Verification items for the finished model (mm, model axes). Face numbers are marked on the shaded views. A direction names the side the tool comes from. Round coordinates to 2 decimals unless told otherwise and drop trailing zeros. Write each loop counter-clockwise with the first axis right and the second up, starting at its lowest first coordinate (ties: lowest second). Pieces come first, ordered by that corner, then holes. Notation, with made-up numbers: M -0.5,28.25 L 42.5,28.25 A10 cw 42.5,47.25 Z; hole C 62.5,54 d1. An arc over 180 degrees is marked long. One line per item, written item: value. Start each with the question number.
Item 1: Gauge pin test, flat ends, axial feed: pin 1 (2 mm diameter, centred on x = -3, y = -4.5, fed in from +Z); pin 2 (2.5 mm diameter, centred on x = -0.5, z = -7.5, fed in from -Y); pin 3 (3 mm diameter, centred on x = -3, z = -7.5, fed in from -Y). Record the tip position at first contact, or that the pin passes through.
Item 2: Section check A-A, the plane y = -8. Record the cut outline in (x, z), then the cut area to 3 significant figures.
Item 3: Section check D-D, the plane y = -9.75. Record the cut outline in (x, z), then the cut area to 3 significant figures.
Item 4: Section check B-B, the plane z = 2. Record the cut outline in (x, y), then the cut area to 3 significant figures.
Item 5: Tool access check on the marked faces 5 and 6. Record the directions out of +Z, -Z, +X, -X, +Y, -Y that give a thin tool (end or side, any length) a straight path to the whole face; none if there is none.
Item 6: Draft check along Y on the marked faces 1, 2, 3 and 4. Enter one of: +Y half, -Y half, draft (parallel to the pull), parting line (faces both ways), or undercut.
Item 7: Thickness scan on probe 1 along Z at (x, y) = (-1, -4.5); probe 2 along Y at (x, z) = (3, -1); probe 3 along Y at (x, z) = (-2.75, -4.5). Record the ranges inside material, lowest first. Write a range as from..to.
Item 8: Section check C-C, the plane x = 1.25. Record the cut outline in (y, z), then the cut area to 3 significant figures.
from build123d import *

# Parameters (mm, degrees)
F1_DEPTH    = 4
F2_T1_DEPTH = 10.764079149
F3_W        = 8
F3_H        = 10
F4_DEPTH    = 7
F5_W        = 8
F5_H        = 2.2
F5_W_2      = 11
F5_H_2      = 2.9
F6_DEPTH    = 25
F7_T1_DEPTH = 18
F7_T3_DEPTH = 17.9874921777
F8_W        = 10.9849025458
F8_H        = 7.8663821071
F9_DEPTH    = 25
F11_DEPTH   = 8
F12_R       = 1


# Not quite as in the source:
# - a fillet or chamfer that OpenCascade refuses, or shapes differently, is made with other operations: its cross-section is extruded or revolved along the edge and cut away or added


with BuildPart() as f1:
    # F0 (on Front) → F1 (new body)
    with BuildSketch(Plane.XZ):
        with BuildLine():
            Line((-1.02606043, 2.8190778624), (-1.3680805733, 3.7587704831))
            ThreePointArc((-1.3680805733, 3.7587704831), (-3.2766081772, 2.2943057454), (-4, 0))
            Line((-4, 0), (-4, -8))
            Line((-4, -8), (-4, -13))
            Line((-4, -13), (4, -13))
            Line((4, -13), (4, -3))
            Line((4, -3), (4, 0))
            ThreePointArc((4, 0), (3.2766081772, 2.2943057454), (1.3680805733, 3.7587704831))
            Line((1.3680805733, 3.7587704831), (1.02606043, 2.8190778624))
            ThreePointArc((1.02606043, 2.8190778624), (0, -3), (-1.02606043, 2.8190778624))
        make_face()
    extrude(amount=F1_DEPTH)

    # F2: fillet of radius 1 on 2 edges, made by hand

    # F2_s2 → F2_t1 (cut)
    with BuildSketch(Plane.XZ.offset(-3.3820395745)):
        with BuildLine():
            ThreePointArc((-2.5427622285, 3.087775939), (-1.6437981614, 3.280553188), (-0.9673790506, 2.6578520976))
            Line((-0.9673790506, 2.6578520976), (-1.3680805733, 3.7587704831))
            ThreePointArc((-1.3680805733, 3.7587704831), (-1.9839937688, 3.4732936423), (-2.5427622285, 3.087775939))
        make_face()
        with BuildLine():
            ThreePointArc((2.5427622285, 3.087775939), (1.6437981614, 3.280553188), (0.9673790506, 2.6578520976))
            Line((0.9673790506, 2.6578520976), (1.3680805733, 3.7587704831))
            ThreePointArc((1.3680805733, 3.7587704831), (1.9839937688, 3.4732936423), (2.5427622285, 3.087775939))
        make_face()
    extrude(amount=F2_T1_DEPTH, mode=Mode.SUBTRACT)

    # F3 (on face) → F4 (join)
    with BuildSketch(Plane.XZ.offset(4)):
        with Locations((0, -8)):
            Rectangle(F3_W, F3_H)
    extrude(amount=F4_DEPTH)

    # F5 (on face) → F6 (cut)
    with BuildSketch(Plane.YZ.offset(4)):
        with Locations((-7, -7.1)):
            Rectangle(F5_W, F5_H)
        with Locations((-5.5, -11.55)):
            Rectangle(F5_W_2, F5_H_2)
    extrude(amount=-F6_DEPTH, mode=Mode.SUBTRACT)

    # F7: fillet of radius 2 on 4 edges, made by hand

    # F7_s2 → F7_t1 (cut)
    with BuildSketch(Plane.YZ.offset(-9)):
        with BuildLine():
            ThreePointArc((-11, -4), (-10.4142135624, -5.4142135624), (-9, -6))
            Line((-9, -6), (-11, -6))
            Line((-11, -6), (-11, -4))
        make_face()
        with BuildLine():
            ThreePointArc((-9, -3), (-10.4142135624, -3.5857864376), (-11, -5))
            Line((-11, -5), (-11, -3))
            Line((-11, -3), (-9, -3))
        make_face()
        with BuildLine():
            ThreePointArc((0, -8.1), (-0.5857864376, -9.5142135624), (-2, -10.1))
            Line((-2, -10.1), (0, -10.1))
            Line((0, -10.1), (0, -8.1))
        make_face()
    extrude(amount=F7_T1_DEPTH, mode=Mode.SUBTRACT)

    # F7_s4 → F7_t3 (cut)
    with BuildSketch(Plane.YZ.offset(-8.9937460889)):
        with BuildLine():
            ThreePointArc((-9.0025015645, -8.2), (-10.3809064397, -8.7508623254), (-11, -10.1))
            Line((-11, -10.1), (-11, -8.2))
            Line((-11, -8.2), (-9.0025015645, -8.2))
        make_face()
    extrude(amount=F7_T3_DEPTH, mode=Mode.SUBTRACT)

    # F8 (on face) → F9 (cut)
    with BuildSketch(Plane.XZ.offset(4)):
        with Locations((-1.4924512729, 0.9331910536)):
            Rectangle(F8_W, F8_H)
    extrude(amount=-F9_DEPTH, mode=Mode.SUBTRACT)

    # F10 (on face) → F11 (join, through all)
    with BuildSketch(Plane.YZ.offset(4)):
        with BuildLine():
            ThreePointArc((-2.3786796564, 2.1213203436), (-1.7283614025, -1.1480502971), (-4.5, -3))
            Line((-4.5, -3), (-9.1097722286, -3))
            ThreePointArc((-9.1097722286, -3), (-1.0366594684, -4.2726189114), (-0.6109127035, 3.8890872965))
            Line((-0.6109127035, 3.8890872965), (-2.3786796564, 2.1213203436))
        make_face()
        with BuildLine():
            Line((-9.1097722286, -3), (-4.5, -3))
            ThreePointArc((-4.5, -3), (-7.2716385975, -1.1480502971), (-6.6213203436, 2.1213203436))
            Line((-6.6213203436, 2.1213203436), (-8.3890872965, 3.8890872965))
            ThreePointArc((-8.3890872965, 3.8890872965), (-9.9701493811, 0.5722462303), (-9.1097722286, -3))
        make_face()
    extrude(amount=-F11_DEPTH)

    # F12
    f12_edges = [f1.edges().sort_by_distance(p)[0] for p in [
        (0, -2.37868, 2.12132),
        (0, -6.62132, 2.12132),
    ]]
    fillet(f12_edges, radius=F12_R)


solid = f1.part
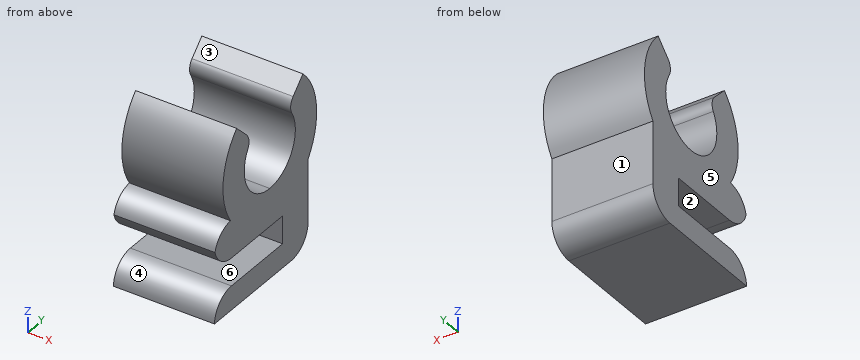
Response values:
1. pin 1: stops at z = -2.83
1. pin 2: stops at y = -10.38
1. pin 3: stops at y = -10.6
2. outline: M -4,-10.1 L 4,-10.1 L 4,-8.2 L -4,-8.2 Z; M -4,-6 L 4,-6 L 4,3.5 L -4,3.5 Z
2. area: 91.2 mm2
3. outline: M -4,-10.1 L 4,-10.1 L 4,-8.34 L -4,-8.34 Z; M -4,-5.85 L 4,-5.85 L 4,-3.15 L -4,-3.15 Z; M -4,-1.64 L 4,-1.64 L 4,1.64 L -4,1.64 Z
3. area: 61.9 mm2
4. outline: M -4,-9.62 L 4,-9.62 L 4,-6.95 L -4,-6.95 Z; M -4,-2.05 L 4,-2.05 L 4,0.62 L -4,0.62 Z
4. area: 42.8 mm2
5. face 5: +Z, -Z, -X, +Y, -Y
5. face 6: +X, -X, -Y
6. face 1: +Y half
6. face 2: draft
6. face 3: undercut
6. face 4: -Y half
7. probe 1: z = -10.1..-8.2, -6..-3
7. probe 2: y = -9.91..-7.33, -1.67..0.91
7. probe 3: y = -10.94..0
8. outline: M -11,-10.1 L -2,-10.1 A2 ccw 0,-8.1 L 0,-3.16 A5.5 ccw -0.61,3.89 L -1.76,2.74 A1 ccw -1.92,1.52 A3 cw long -7.08,1.52 A1 ccw -7.24,2.74 L -8.39,3.89 A5.5 ccw -9.11,-3 A2 ccw -10.94,-4.5 A2 ccw -9,-6 L -3,-6 L -3,-8.2 L -9,-8.2 A2 ccw Z
8. area: 90.7 mm2
